Read the model definition and answer for the solid it produces. Units are mm, in the model's axes. Give positions to 0.01 mm unless a question says otherwise; leave off trailing zeros. Write each loop counter-clockwise with the first axis right and the second up, starting at its lowest first coordinate (ties: lowest second). Pieces come first, ordered by that corner, then holes. Notation, with made-up numbers: M 32.25,66 L 72.25,66 A19 cw 72.25,72 Z; hole C 81.5,85.5 d3. An arc over 180 degrees is marked long. Answer as CSV lines item,"result". Start each with the question number.
```python
from build123d import *

# Parameters (mm, degrees)
SKETCH1_W               = 825.5
SKETCH1_H               = 1016
BOSS_EXTRUDE1_DEPTH     = 6.35
CAVITY1_START           = -69.750581005
CAVITY1_OUTLINE_R       = 12.7
CAVITY1_DEPTH           = 25.186721765
CAVITY1_2_OUTLINE_R     = 12.7
CAVITY1_2_DEPTH         = 25.186721765
CAVITY1_START_2         = 64.130873345
CAVITY1_3_OUTLINE_R     = 12.7
CAVITY1_3_DEPTH         = 25.120529807
CAVITY1_4_OUTLINE_R     = 12.7
CAVITY1_4_DEPTH         = 25.120529807
CAVITY1_START_3         = -292.036063147
CAVITY1_5_OUTLINE_R     = 12.7
CAVITY1_5_DEPTH         = 24.516904948
CAVITY1_6_OUTLINE_R     = 12.7
CAVITY1_6_DEPTH         = 24.516904948
CAVITY1_START_4         = 116.389417883
CAVITY1_7_OUTLINE_R     = 12.7
CAVITY1_7_DEPTH         = 16.544031778
CAVITY1_8_OUTLINE_R     = 12.7
CAVITY1_8_DEPTH         = 16.544031778
CAVITY1_START_5         = 111.910581246
CAVITY1_9_OUTLINE_R     = 12.7
CAVITY1_9_DEPTH         = 18.901264253
CAVITY1_START_6         = -6.35
CAVITY1_10_OUTLINE_R    = 12.7
CAVITY1_10_DEPTH        = 12.7
CAVITY1_11_OUTLINE_R    = 12.7
CAVITY1_11_DEPTH        = 18.901264253
CUT_EXTRUDE4_DEPTH      = 1097.658052904
CUT_EXTRUDE4_DEPTH_BACK = 1097.658052904
SKETCH5_W               = 12.7
SKETCH5_H               = 508
CUT_EXTRUDE5_DEPTH      = 1097.658052904
CUT_EXTRUDE5_DEPTH_BACK = 1097.658052904
SKETCH6_W               = 12.7
SKETCH6_H               = 508
SKETCH7_W               = 127
SKETCH7_H               = 12.7
CUT_EXTRUDE6_DEPTH      = 1097.658052904
SKETCH8_W               = 127
SKETCH8_H               = 12.7
CUT_EXTRUDE7_DEPTH      = 1097.658052904


# Read off the part's stored shape, not the designer's step: Cavity1
with BuildPart() as part:
    # Sketch1 → Boss-Extrude1 (new, symmetric)
    with BuildSketch(Plane(origin=(0, 0, 0), x_dir=(0, 0, -1), z_dir=(1, 0, 0))):
        with Locations((0, 508)):
            Rectangle(SKETCH1_W, SKETCH1_H)
    extrude(amount=BOSS_EXTRUDE1_DEPTH, both=True)

    # Cavity1 outline → Cavity1 (cut)
    with BuildSketch(Plane(origin=(0, 0, 0), x_dir=(0, 1, 0), z_dir=(0.9138115486202553, 0, 0.4061384660534521)).offset(CAVITY1_START)):
        with Locations((469.9, -128.603745276)):
            Circle(CAVITY1_OUTLINE_R)
    extrude(amount=CAVITY1_DEPTH, mode=Mode.SUBTRACT)

    # Cavity1 2 outline → Cavity1 2 (cut)
    with BuildSketch(Plane(origin=(0, 0, 0), x_dir=(0, 1, 0), z_dir=(0.913811548620257, 0, -0.406138466053448)).offset(CAVITY1_START)):
        with Locations((469.9, 128.603745276)):
            Circle(CAVITY1_2_OUTLINE_R)
    extrude(amount=CAVITY1_2_DEPTH, mode=Mode.SUBTRACT)

    # Cavity1 3 outline → Cavity1 3 (cut)
    with BuildSketch(Plane(origin=(0, 0, 0), x_dir=(-0.14398491314217557, 0.9878322579058099, -0.05878584037121407), z_dir=(0.9145455226247352, 0.15552308587701602, 0.37338861365384507)).offset(CAVITY1_START_2)):
        with Locations((840.881224499, -134.757426505)):
            Circle(CAVITY1_3_OUTLINE_R)
    extrude(amount=CAVITY1_3_DEPTH, mode=Mode.SUBTRACT)

    # Cavity1 4 outline → Cavity1 4 (cut)
    with BuildSketch(Plane(origin=(0, 0, 0), x_dir=(-0.14398491314217668, 0.9878322579058096, 0.05878584037121399), z_dir=(0.9145455226247362, 0.15552308587701702, -0.37338861365384207)).offset(CAVITY1_START_2)):
        with Locations((840.881224499, 134.757426505)):
            Circle(CAVITY1_4_OUTLINE_R)
    extrude(amount=CAVITY1_4_DEPTH, mode=Mode.SUBTRACT)

    # Cavity1 5 outline → Cavity1 5 (cut)
    with BuildSketch(Plane(origin=(0, 0, 0), x_dir=(0.3827993278239342, 0.9234408320803411, 0.026864554050110373), z_dir=(0.9211751685610859, -0.38374083656390695, 0.0646473447226402)).offset(CAVITY1_START_3)):
        with Locations((711.455758667, 208.844736372)):
            Circle(CAVITY1_5_OUTLINE_R)
    extrude(amount=CAVITY1_5_DEPTH, mode=Mode.SUBTRACT)

    # Cavity1 6 outline → Cavity1 6 (cut)
    with BuildSketch(Plane(origin=(0, 0, 0), x_dir=(0.3827993278239134, 0.9234408320803503, -0.02686455405009277), z_dir=(0.9211751685610978, -0.3837408365638849, -0.06464734472260218)).offset(CAVITY1_START_3)):
        with Locations((711.455758667, -208.844736372)):
            Circle(CAVITY1_6_OUTLINE_R)
    extrude(amount=CAVITY1_6_DEPTH, mode=Mode.SUBTRACT)

    # Cavity1 7 outline → Cavity1 7 (cut)
    with BuildSketch(Plane(origin=(0, 0, 0), x_dir=(-0.14162907065889588, 0.989911458049715, -0.00406344265182396), z_dir=(0.9895042824022925, 0.14168735025360304, 0.028389608761606212)).offset(CAVITY1_START_4)):
        with Locations((829.701952497, 203.742071242)):
            Circle(CAVITY1_7_OUTLINE_R)
    extrude(amount=CAVITY1_7_DEPTH, mode=Mode.SUBTRACT)

    # Cavity1 8 outline → Cavity1 8 (cut)
    with BuildSketch(Plane(origin=(0, 0, 0), x_dir=(-0.1416290706588989, 0.9899114580497147, 0.00406344265182273), z_dir=(0.9895042824022923, 0.14168735025360601, -0.028389608761597008)).offset(CAVITY1_START_4)):
        with Locations((829.701952497, -203.742071242)):
            Circle(CAVITY1_8_OUTLINE_R)
    extrude(amount=CAVITY1_8_DEPTH, mode=Mode.SUBTRACT)

    # Cavity1 9 outline → Cavity1 9 (cut)
    with BuildSketch(Plane(origin=(0, 0, 0), x_dir=(-0.2138887427613121, 0.9767426935099688, 0.015010542790871387), z_dir=(0.9743462537907107, 0.21441480983106392, -0.06837884942814358)).offset(CAVITY1_START_5)):
        with Locations((484.491346969, -208.844736372)):
            Circle(CAVITY1_9_OUTLINE_R)
    extrude(amount=CAVITY1_9_DEPTH, mode=Mode.SUBTRACT)

    # Cavity1 10 outline → Cavity1 10 (cut)
    with BuildSketch(Plane.YZ.offset(CAVITY1_START_6)):
        with Locations((469.9, -200)):
            Circle(CAVITY1_10_OUTLINE_R)
        with Locations((469.9, 200)):
            Circle(CAVITY1_10_OUTLINE_R)
    extrude(amount=CAVITY1_10_DEPTH, mode=Mode.SUBTRACT)

    # Cavity1 11 outline → Cavity1 11 (cut)
    with BuildSketch(Plane(origin=(0, 0, 0), x_dir=(-0.21388874276128378, 0.9767426935099748, -0.015010542790877034), z_dir=(0.9743462537907144, 0.21441480983103609, 0.06837884942817862)).offset(CAVITY1_START_5)):
        with Locations((484.491346969, 208.844736372)):
            Circle(CAVITY1_11_OUTLINE_R)
    extrude(amount=CAVITY1_11_DEPTH, mode=Mode.SUBTRACT)

    # Sketch5 → Cut-Extrude4 (cut, two sides: drawn at the far end of the back side and taken through both)
    with BuildSketch(Plane(origin=(0, 0, 0), x_dir=(0, 0, -1), z_dir=(1, 0, 0)).offset(-CUT_EXTRUDE4_DEPTH_BACK)):
        with Locations((76.2, 254)):
            Rectangle(SKETCH5_W, SKETCH5_H)
    extrude(amount=CUT_EXTRUDE4_DEPTH + CUT_EXTRUDE4_DEPTH_BACK, mode=Mode.SUBTRACT)

    # Sketch6 → Cut-Extrude5 (cut, two sides: drawn at the far end of the back side and taken through both)
    with BuildSketch(Plane(origin=(0, 0, 0), x_dir=(0, 0, -1), z_dir=(1, 0, 0)).offset(-CUT_EXTRUDE5_DEPTH_BACK)):
        with Locations((-76.2, 254)):
            Rectangle(SKETCH6_W, SKETCH6_H)
    extrude(amount=CUT_EXTRUDE5_DEPTH + CUT_EXTRUDE5_DEPTH_BACK, mode=Mode.SUBTRACT)

    # Sketch7 → Cut-Extrude6 (cut, symmetric)
    with BuildSketch(Plane(origin=(0, 0, 0), x_dir=(0, 0, -1), z_dir=(1, 0, 0))):
        with Locations((349.25, 704.85)):
            Rectangle(SKETCH7_W, SKETCH7_H)
    cut_extrude6 = extrude(amount=CUT_EXTRUDE6_DEPTH, both=True, mode=Mode.SUBTRACT)

    # Sketch8 → Cut-Extrude7 (cut, symmetric)
    with BuildSketch(Plane(origin=(0, 0, 0), x_dir=(0, 0, -1), z_dir=(1, 0, 0))):
        with Locations((-349.25, 539.75)):
            Rectangle(SKETCH8_W, SKETCH8_H)
    cut_extrude7 = extrude(amount=CUT_EXTRUDE7_DEPTH, both=True, mode=Mode.SUBTRACT)

    # Mirror1: Cut-Extrude6, Cut-Extrude7 across plane
    add(cut_extrude6.mirror(Plane.XY), mode=Mode.SUBTRACT)
    add(cut_extrude7.mirror(Plane.XY), mode=Mode.SUBTRACT)


solid = part.part
```
1. Given pin 1 (6.5 mm diameter, centred on x = 1, y = 539, fed in from +Z); pin 2 (20.5 mm diameter, centred on y = 469.9, z = 200, fed in from +X), each flat-ended and moving along its own axis, determine where each tip first touches the part or whether it passes through.
2. Find section A-A on z = -341. Determine the outline of the cut face in (x, y), then the cut area to 3 significant figures.
3. Determine the mould class of faces 1 (the face through (1.7, 826.42, -203.32)), 2 (the face through (6.35, 515, 6)) for opening direction Z: +Z half, -Z half, draft (parallel to the pull), parting line (faces both ways), or undercut.
4. Find section B-B on y = 391. Determine the outline of the cut face in (x, z).
5. Find section C-C on x = 0.5. State how many separate pieces and enclosed holes the cut face has, then the cut area to 3 significant figures.
6. Find the intervals of material crossed by line 1 (Z direction, x = 0, y = 42); line 2 (Y direction, x = -6, z = 321); line 3 (Z direction, x = -3.5, y = 850), in increasing order. Write a range as [from, to].
Computed:
1,pin 1,"stops at z = 285.75"
1,pin 2,"passes through"
2,outline,"M -6.35,0 L 6.35,0 L 6.35,533.4 L -6.35,533.4 Z; M -6.35,546.1 L 6.35,546.1 L 6.35,698.5 L -6.35,698.5 Z; M -6.35,711.2 L 6.35,711.2 L 6.35,1016 L -6.35,1016 Z"
2,area,"12,600 mm^2"
3,face 1,"undercut"
3,face 2,"draft"
4,outline,"M -6.35,-412.75 L 6.35,-412.75 L 6.35,-82.55 L -6.35,-82.55 Z; M -6.35,-69.85 L 6.35,-69.85 L 6.35,69.85 L -6.35,69.85 Z; M -6.35,82.55 L 6.35,82.55 L 6.35,412.75 L -6.35,412.75 Z"
5,separate pieces,"1"
5,enclosed holes,"12"
5,area,"813,000 mm^2"
6,line 1,"z = [-412.75, -82.55], [-69.85, 69.85], [82.55, 412.75]"
6,line 2,"y = [0, 533.4], [546.1, 698.5], [711.2, 1016]"
6,line 3,"z = [-412.75, -209.39], [-198.15, -157.16], [-135.73, 135.73], [157.16, 198.15], [209.39, 412.75]"
